Can you work these out from the model? Positions are in its coordinate system, mm. Coordinates: 2 decimals unless noted, no trailing zeros. Loops run counter-clockwise (first coordinate to the right, second up) from the corner with the lowest first, then second, coordinate; pieces in that order, holes last. Notation, with made-up numbers: M -25.5,-27.75 L -6.5,-27.75 A19 cw -6.5,-17.75 Z; hole C 85,81 d2. An arc over 180 degrees is marked long. Answer as a JSON object with one key per item and string values. Group by question number.
Item 1: We'd pull the mould along X, two halves only. Please class faces 1 (the cylindrical face through (-26.49, 0.99, -28.61)), 2 (the flat face through (0, 1, -32.5)), 3 (the cylindrical face through (31.99, 1.01, -29.65)): +X half, -X half, draft (parallel to the pull), parting line (faces both ways), or undercut.
Item 2: If I drill on line 1 (X direction, y = 0.9, z = 27.5); line 2 (Z direction, x = 27.5, y = 1.8); line 3 (Z direction, x = 0, y = 0.65), over which ranges is the centre line in solid material (lowest first)?
Item 3: Suppose I cut it at A-A (z = -18). Write out the boundary of the cut face in (x, y), then the cut area to 3 significant figures.
Item 4: Suppose I cut it at C-C (x = -27.5). Write out the boundary of the cut face in (y, z).
Item 5: Suppose I cut it at D-D (x = -2.5). Write out the boundary of the cut face in (y, z).
Item 6: Suppose I cut it at B-B (y = 0.3). Write out the boundary of the cut face in (x, z), then the cut area to 3 significant figures.
```python
from build123d import *

# Parameters (mm, degrees)
SKETCH_1_W          = 70
SKETCH_1_H          = 65
SKETCH_1_R          = 22.5
SKETCH_1_R_2        = 1.5
EXTRUDE_1_DEPTH     = 10
FILLET_1_R          = 10
FILLET_2_R          = 10
FILLET_3_R          = 10
FILLET_4_R          = 10
SKETCH_2_W          = 161.633033244
SKETCH_2_H          = 138.385284329
CUT_EXTRUDE_1_DEPTH = 8


with BuildPart() as part:
    # 草图1 → 凸台-拉伸1 (new body)
    with BuildSketch(Plane(origin=(0, 0, 0), x_dir=(1, 0, 0), z_dir=(0, 1, 0))):
        Rectangle(SKETCH_1_W, SKETCH_1_H)
        with Locations(Location((0, 0, 0), (0, 0, 270))):
            Circle(SKETCH_1_R, mode=Mode.SUBTRACT)
        with Locations(Location((-27.5, 27.5, 0), (0, 0, 270))):
            Circle(SKETCH_1_R_2, mode=Mode.SUBTRACT)
        with Locations(Location((-27.5, -27.5, 0), (0, 0, 270))):
            Circle(SKETCH_1_R_2, mode=Mode.SUBTRACT)
        with Locations(Location((27.5, -27.5, 0), (0, 0, 270))):
            Circle(SKETCH_1_R_2, mode=Mode.SUBTRACT)
        with Locations(Location((27.5, 27.5, 0), (0, 0, 270))):
            Circle(SKETCH_1_R_2, mode=Mode.SUBTRACT)
    extrude(amount=EXTRUDE_1_DEPTH)

    # 圆角1
    fillet_1_edges = [part.edges().sort_by_distance(p)[0] for p in [
        (-35, 5, -32.5),
    ]]
    fillet(fillet_1_edges, radius=FILLET_1_R)

    # 圆角2
    fillet_2_edges = [part.edges().sort_by_distance(p)[0] for p in [
        (35, 5, -32.5),
    ]]
    fillet(fillet_2_edges, radius=FILLET_2_R)

    # 圆角3
    fillet_3_edges = [part.edges().sort_by_distance(p)[0] for p in [
        (-35, 5, 32.5),
    ]]
    fillet(fillet_3_edges, radius=FILLET_3_R)

    # 圆角4
    fillet_4_edges = [part.edges().sort_by_distance(p)[0] for p in [
        (35, 5, 32.5),
    ]]
    fillet(fillet_4_edges, radius=FILLET_4_R)

    # 草图2 → 切除-拉伸1 (cut)
    with BuildSketch(Plane(origin=(0, 10, 0), x_dir=(1, 0, 0), z_dir=(0, 1, 0))):
        with Locations((-39.612940585, 34.19866222)):
            Rectangle(SKETCH_2_W, SKETCH_2_H)
    extrude(amount=-CUT_EXTRUDE_1_DEPTH, mode=Mode.SUBTRACT)


solid = part.part
```
From the geometry:
{
 "1": {"face 1": "undercut", "face 2": "draft", "face 3": "+X half"},
 "2": {"line 1": "-33.66 to -29, -26 to 26, 29 to 33.66", "line 2": "-32.18 to -29, -26 to 26, 29 to 32.18", "line 3": "-32.5 to -22.5, 22.5 to 32.5"},
 "3": {"outline": "M -35,0 L -13.5,0 L -13.5,2 L -35,2 Z; M 13.5,0 L 35,0 L 35,2 L 13.5,2 Z", "area": "86.0 mm2"},
 "4": {"outline": "M 0,-32.18 L 2,-32.18 L 2,-29 L 0,-29 Z; M 0,-26 L 2,-26 L 2,26 L 0,26 Z; M 0,29 L 2,29 L 2,32.18 L 0,32.18 Z"},
 "5": {"outline": "M 0,-32.5 L 2,-32.5 L 2,-22.36 L 0,-22.36 Z; M 0,22.36 L 2,22.36 L 2,32.5 L 0,32.5 Z"},
 "6": {"outline": "M -35,-22.5 A10 ccw -25,-32.5 L 25,-32.5 A10 ccw 35,-22.5 L 35,22.5 A10 ccw 25,32.5 L -25,32.5 A10 ccw -35,22.5 Z; hole C -27.5,-27.5 d3; hole C -27.5,27.5 d3; hole C 0,0 d45; hole C 27.5,-27.5 d3; hole C 27.5,27.5 d3", "area": "2,850 mm2"}
}
